Here's how the part is built. I have some questions about the finished solid (model axes, mm). A direction names the side the tool comes from. Round coordinates to 2 decimals unless told otherwise and drop trailing zeros. Order: outer loops, then holes, each group sorted by start corner. A loop starts at its lowest first (then second) coordinate and runs counter-clockwise, first axis right, second up.
```python
from build123d import *

# Parameters (mm, degrees)
SKETCH1_W           = 142.755639788
SKETCH1_H           = 271.365530146
BOSS_EXTRUDE1_DEPTH = 12.7
HOLE1_D             = 3.175
HOLE1_DEPTH         = 31.75
HOLE1_CSINK_D       = 10.16
HOLE1_CSINK_ANGLE   = 82
HOLE1_TIP           = 0.953866233
SKETCH4_W           = 79.255639788
SKETCH4_H           = 106.265530146
CUT_EXTRUDE1_DEPTH  = 302.349406056
FILLET1_R           = 31.75


with BuildPart() as part:
    # Sketch1 → Boss-Extrude1 (new body)
    with BuildSketch(Plane.XY):
        with Locations((-163.375147287, -52.841023691)):
            Rectangle(SKETCH1_W, SKETCH1_H)
    extrude(amount=BOSS_EXTRUDE1_DEPTH)

    # Hole1
    with Locations(Plane(origin=(181.039434513, -52.974999997, 0), x_dir=(0, -1, 0), z_dir=(0, 0, -1))):
        with Locations((129.198788767, 384.042401694), (-129.466741379, 384.042401694), (-129.466741379, 304.786761906), (-110.416741379, 409.442401694), (-0.133976306, 409.442401694), (110.148788767, 409.442401694), (129.198788767, 304.786761906)):
            CounterSinkHole(HOLE1_D / 2, HOLE1_CSINK_D / 2, depth=HOLE1_DEPTH, counter_sink_angle=HOLE1_CSINK_ANGLE)
            with Locations((0, 0, -(HOLE1_DEPTH + HOLE1_TIP / 2))):  # 118° drill point
                Cone(0, HOLE1_D / 2, HOLE1_TIP, mode=Mode.SUBTRACT)

    # Sketch4 → Cut-Extrude1 (cut, through all)
    with BuildSketch(Plane.XY.offset(12.7)):
        with Locations((-163.375147287, -52.841023691)):
            Rectangle(SKETCH4_W, SKETCH4_H)
    extrude(amount=-CUT_EXTRUDE1_DEPTH, mode=Mode.SUBTRACT)

    # Fillet1
    fillet1_edges = [part.edges().sort_by_distance(p)[0] for p in [
        (-203.002967181, -105.973788764, 6.35),
        (-203.002967181, 0.291741382, 6.35),
        (-123.747327393, 0.291741382, 6.35),
        (-123.747327393, -105.973788764, 6.35),
    ]]
    fillet(fillet1_edges, radius=FILLET1_R)


solid = part.part
```
1. If we section it at B-B, the plane x = -181: Write out the boundary of the cut face in (y, z), and give its area (3 significant figures).
Evaluation:
outline: (-188.52, 0) - (-104.44, 0) - (-104.44, 12.7) - (-188.52, 12.7) - close; (-1.24, 0) - (82.84, 0) - (82.84, 12.7) - (-1.24, 12.7) - close
area: 2,140 mm2
2. If we section it at A-A, the plane y = -43.5: Write out the boundary of the cut face in (x, z).
Evaluation:
outline: (-234.75, 0) - (-203, 0) - (-203, 12.7) - (-234.75, 12.7) - close; (-123.75, 0) - (-92, 0) - (-92, 12.7) - (-123.75, 12.7) - close
3. If we section it at C-C, the plane z = 7.75: State how many separate pieces and enclosed holes the cut face has, and give its area (3 significant figures).
Evaluation:
separate pieces: 1
enclosed holes: 8
area: 31,100 mm2
4. If we mould it in two halves opening along X, with no side actions, what happens to faces 1 (the flat face through (-164, -188.524, 6)), 2 (the cylindrical face through (-132.801, -9.256, 6.261)), 3 (the flat face through (-91.997, -55, 6))? For each: released by +X, released by -X, zero draft, split by the parting line, or undercut.
Evaluation:
face 1: zero draft
face 2: undercut
face 3: released by +X
5. I need wall thicknesses on probe 1 along Y at (x, z) = (-167, 10); probe 2 along X at (y, z) = (-70, 7); probe 3 along X at (y, z) = (-87, 9.25). Which ranges of each line are inside material? Lowest first, please.
Evaluation:
probe 1: y = -188.52 to -105.97, 0.29 to 82.84
probe 2: x = -234.75 to -203, -123.75 to -92
probe 3: x = -234.75 to -200.32, -126.43 to -92
6. I'm going to push flat-ended pins straight in: P1, Ø1.9, axis at x = -228.4, y = -52.84, coming from the +Z side; P2, Ø5, axis at x = -203, y = -182.17, coming from the -Z side. Where does each tip first touch, or does it pass through?
Evaluation:
P1: passes through
P2: stops at z = 2.96
7. On a 3-axis mill with a long thin cutter (end or side, diameter ignored), from which of +Z, -Z, +X, -X, +Y, -Y can I reach the whole of each face in a straight line? I mean faces 4 (the cylindrical face through (-193.455, -8.762, 6.261)), 5 (the flat face through (-164, 82.842, 6)). Say none if no direction works.
Evaluation:
face 4: +Z, -Z
face 5: +Z, -Z, +X, -X, +Y
